Read the model definition and answer for the solid it produces. Units are mm, in the model's axes. Give positions to 0.01 mm unless a question says otherwise; leave off trailing zeros. Order: outer loops, then holes, each group sorted by start corner. A loop starts at its lowest first (then second) coordinate and runs counter-clockwise, first axis right, second up. Notation, with made-up numbers: (-13.5, 44.5) - (28.5, 44.5) arc R27 cw to (28.5, 75.5) - close; hole circle Ø8 at (28.25, 72). An arc over 180 degrees is marked (long way). Return JSON: item names as keys, results as strings.
```python
from build123d import *

# Parameters (mm, degrees)
SKETCH1_R           = 2.1
SKETCH1_R_2         = 11
SKETCH1_R_3         = 1.6
BOSS_EXTRUDE1_DEPTH = 1.5


with BuildPart() as part:
    # Sketch1 → Boss-Extrude1 (new body, symmetric)
    with BuildSketch(Plane.XY):
        with BuildLine():
            Line((107, -145), (107, -110.895624471))
            ThreePointArc((107, -110.895624471), (105.553363517, -102.514749396), (101.380874638, -95.103800692))
            Line((101.380874638, -95.103800692), (46.619125362, -27.896199308))
            ThreePointArc((46.619125362, -27.896199308), (42.446636483, -20.485250604), (41, -12.104375529))
            Line((41, -12.104375529), (41, 154))
            ThreePointArc((41, 154), (39.535533906, 157.535533906), (36, 159))
            Line((36, 159), (-36, 159))
            ThreePointArc((-36, 159), (-39.535533906, 157.535533906), (-41, 154))
            Line((-41, 154), (-41, -61.522167809))
            ThreePointArc((-41, -61.522167809), (-39.376465331, -70.384496434), (-34.716730508, -78.095761236))
            Line((-34.716730508, -78.095761236), (10.716730508, -129.404238764))
            ThreePointArc((10.716730508, -129.404238764), (15.198642313, -136.659946441), (16.980869565, -145))
            ThreePointArc((16.980869565, -145), (18.445335659, -148.535533906), (21.980869565, -150))
            Line((21.980869565, -150), (102, -150))
            ThreePointArc((102, -150), (105.535533906, -148.535533906), (107, -145))
        make_face()
        with Locations((96, -107)):
            Circle(SKETCH1_R, mode=Mode.SUBTRACT)
        with Locations((96, -131)):
            Circle(SKETCH1_R, mode=Mode.SUBTRACT)
        with Locations((78, -107)):
            Circle(SKETCH1_R, mode=Mode.SUBTRACT)
        with Locations((78, -131)):
            Circle(SKETCH1_R, mode=Mode.SUBTRACT)
        with Locations((46, -107)):
            Circle(SKETCH1_R, mode=Mode.SUBTRACT)
        with Locations((46, -131)):
            Circle(SKETCH1_R, mode=Mode.SUBTRACT)
        with Locations((28, -107)):
            Circle(SKETCH1_R, mode=Mode.SUBTRACT)
        with Locations((28, -131)):
            Circle(SKETCH1_R, mode=Mode.SUBTRACT)
        with Locations((51, -143)):
            Circle(SKETCH1_R, mode=Mode.SUBTRACT)
        with Locations((73, -143)):
            Circle(SKETCH1_R, mode=Mode.SUBTRACT)
        with Locations((0, 126)):
            Circle(SKETCH1_R, mode=Mode.SUBTRACT)
        Circle(SKETCH1_R, mode=Mode.SUBTRACT)
        with Locations((-32.666666667, 144)):
            Circle(SKETCH1_R, mode=Mode.SUBTRACT)
        with Locations((-17.333333333, 124)):
            Circle(SKETCH1_R, mode=Mode.SUBTRACT)
        with Locations((-17.333333333, -31)):
            Circle(SKETCH1_R, mode=Mode.SUBTRACT)
        with Locations((-32.666666667, -51)):
            Circle(SKETCH1_R, mode=Mode.SUBTRACT)
        with Locations((-6.5, 63)):
            Circle(SKETCH1_R_2, mode=Mode.SUBTRACT)
        with Locations((-22, 78.5)):
            Circle(SKETCH1_R_3, mode=Mode.SUBTRACT)
        with Locations((9, 78.5)):
            Circle(SKETCH1_R_3, mode=Mode.SUBTRACT)
        with Locations((-22, 47.5)):
            Circle(SKETCH1_R_3, mode=Mode.SUBTRACT)
        with Locations((9, 47.5)):
            Circle(SKETCH1_R_3, mode=Mode.SUBTRACT)
    extrude(amount=BOSS_EXTRUDE1_DEPTH, both=True)


solid = part.part
```
Q1. A cutting plane is placed at A-A (x = -6.5). Write down the section's boundary in (y, z), and give its area (3 significant figures).
Values:
{"outline": "(-109.96, -1.5) - (52, -1.5) - (52, 1.5) - (-109.96, 1.5) - close; (74, -1.5) - (159, -1.5) - (159, 1.5) - (74, 1.5) - close", "area": "741 mm²"}
Q2. Determine the mould class of faces 1 (the cylindrical face through (15.154, -136.549, 0.021)), 2 (the cylindrical face through (42.487, -20.598, 0.021)), 3 (the cylindrical face through (-7.932, 73.906, -0.021)), 4 (the flat face through (16, 7, 1.5)) for opening direction X: released by +X, released by -X, zero draft, split by the parting line, or undercut.
Values:
{"face 1": "released by -X", "face 2": "released by +X", "face 3": "undercut", "face 4": "zero draft"}
Q3. A cutting plane is placed at B-B (y = 68). Write down the section's boundary in (x, z), and give its area (3 significant figures).
Values:
{"outline": "(-41, -1.5) - (-16.3, -1.5) - (-16.3, 1.5) - (-41, 1.5) - close; (3.3, -1.5) - (41, -1.5) - (41, 1.5) - (3.3, 1.5) - close", "area": "187 mm²"}
Q4. A cutting plane is placed at D-D (x = 65). Write down the section's boundary in (y, z).
Values:
{"outline": "(-150, -1.5) - (-50.45, -1.5) - (-50.45, 1.5) - (-150, 1.5) - close"}
Q5. Consider L1, parallel to X at y = 47, z = 0.4; L2, parallel to Y at x = 96, z = -0.05; L3, parallel to X at y = 34, z = 0.85. Determine where each line is inside the solid, lowest interval first.
Values:
{"L1": "x = -41 to -23.52, -20.48 to 7.48, 10.52 to 41", "L2": "y = -150 to -133.1, -128.9 to -109.1, -104.9 to -88.5", "L3": "x = -41 to 41"}
Q6. Given pin 1 (0.9 mm diameter, centred on y = 62, z = 0, fed in from +X); pin 2 (5.5 mm diameter, centred on x = 28, y = -107, fed in from +Z), each flat-ended and moving along its own axis, determine where each tip first touches the part or whether it passes through.
Values:
{"pin 1": "stops at x = 41", "pin 2": "stops at z = 1.5"}
Q7. A cutting plane is placed at C-C (z = -0.7). Give the number of separate pieces and of enclosed holes in the cut face, and give its area (3 significant figures).
Values:
{"separate pieces": "1", "enclosed holes": "21", "area": "27,800 mm²"}
